from build123d import *

# Parameters (mm, degrees)
F0_W     = 129.44272
F0_H     = 80
F1_DEPTH = 2
F2_W     = 129.44272
F2_H     = 80
F2_W_2   = 125.44272
F2_H_2   = 76
F3_DEPTH = 2


with BuildPart() as f1:
    # F0 (on Top) → F1 (new body)
    with BuildSketch(Plane.XY):
        Rectangle(F0_W, F0_H)
    extrude(amount=-F1_DEPTH)

    # F2 (on Top) → F3 (join)
    with BuildSketch(Plane.XY):
        Rectangle(F2_W, F2_H)
        Rectangle(F2_W_2, F2_H_2, mode=Mode.SUBTRACT)
    extrude(amount=F3_DEPTH)


solid = f1.part
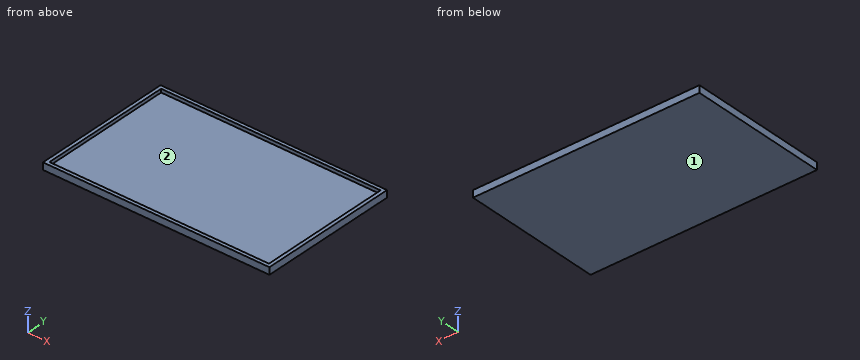
Geometry check sheet. Reference: the model listing, model coordinates, mm. Face numbers are marked on the shaded views. Round coordinates to 2 decimals unless told otherwise and drop trailing zeros. Order: outer loops, then holes, each group sorted by start corner. A loop starts at its lowest first (then second) coordinate and runs counter-clockwise, first axis right, second up. Notation, with made-up numbers: M 27.25,73 L 47.25,73 A29 cw 47.25,105 Z; hole C 1.5,79.5 d4. An arc over 180 degrees is marked long. Answer in a Markdown table with one row per item. Add a question column.
Item 1: Sectioned sample at A-A, the plane z = 0.9. Enter the section's corners in (x, y).
Item 2: Sectioned sample at C-C, the plane x = -37. Enter the section's corners in (y, z).
Item 3: Depth check by flat-ended pin: pin 1 Ø12 at (x, y) = (7, 26) entering from +Z. Enter the tip coordinate at first touch or a pass-through.
Item 4: Sectioned sample at B-B, the plane y = -0.5. Enter the section's corners in (x, z), plus the area to 3 significant figures.
Item 5: Draft check along Y on the marked faces 1 and 2. Enter one of: released by +Y, released by -Y, zero draft, split by the parting line, or undercut.
Item 6: Material ranges on L1, parallel to X at y = 16, z = 1.4; L2, parallel to Y at x = -12, z = 0.4; L3, parallel to Z at x = -14, y = -25, recorded low to high. Write a range as [from, to].
Filled in:
| question | item | result |
|---|---|---|
| 1 | outline | M -64.72,-40 L 64.72,-40 L 64.72,40 L -64.72,40 Z; hole M -62.72,-38 L 62.72,-38 L 62.72,38 L -62.72,38 Z |
| 2 | outline | M -40,-2 L 40,-2 L 40,2 L 38,2 L 38,0 L -38,0 L -38,2 L -40,2 Z |
| 3 | pin 1 | stops at z = 0 |
| 4 | outline | M -64.72,-2 L 64.72,-2 L 64.72,2 L 62.72,2 L 62.72,0 L -62.72,0 L -62.72,2 L -64.72,2 Z |
| 4 | area | 267 mm² |
| 5 | face 1 | zero draft |
| 5 | face 2 | undercut |
| 6 | L1 | x = [-64.72, -62.72], [62.72, 64.72] |
| 6 | L2 | y = [-40, -38], [38, 40] |
| 6 | L3 | z = [-2, 0] |
